```python
from build123d import *
from OCP.BRepFilletAPI import BRepFilletAPI_MakeChamfer

# Parameters (mm, degrees)
SKETCH1_W           = 251
SKETCH1_H           = 24.5
SKETCH1_W_2         = 243
SKETCH1_H_2         = 16.5
BOSS_EXTRUDE1_DEPTH = 25
SKETCH1_2_W         = 251
SKETCH1_2_H         = 24.5
BOSS_EXTRUDE2_DEPTH = 4
CHAMFER1_SIZE       = 10
CHAMFER1_SIZE2      = 1.763269807
FILLET1_R           = 10
FILLET2_R           = 1
FILLET4_R           = 10
FILLET5_R           = 5


with BuildPart() as part:
    # Sketch1 → Boss-Extrude1 (new body)
    with BuildSketch(Plane(origin=(0, 0, 0), x_dir=(1, 0, 0), z_dir=(0, 1, 0))):
        Rectangle(SKETCH1_W, SKETCH1_H)
        Rectangle(SKETCH1_W_2, SKETCH1_H_2, mode=Mode.SUBTRACT)
    extrude(amount=BOSS_EXTRUDE1_DEPTH)

    # Sketch1<2> → Boss-Extrude2 (add)
    with BuildSketch(Plane(origin=(0, 0, 0), x_dir=(1, 0, 0), z_dir=(0, 1, 0))):
        Rectangle(SKETCH1_2_W, SKETCH1_2_H)
    extrude(amount=-BOSS_EXTRUDE2_DEPTH)

    # Chamfer1: one chamfer whose edges measure the first distance from different faces: ONE call of the kernel's chamfer builder (chamfer() names one face for all edges)
    chamfer1_edges_1 = [part.edges().sort_by_distance(p)[0] for p in [
        (121.5, 12.5, 8.25),
        (0, 0, 8.25),
        (-121.5, 12.5, 8.25),
    ]]
    chamfer1_side_1 = [part.faces().sort_by_distance(p)[0] for p in [
        (0, 12.5, 8.25),
    ]]
    chamfer1_edges_2 = [part.edges().sort_by_distance(p)[0] for p in [
        (0, 0, -8.25),
        (121.5, 12.5, -8.25),
        (-121.5, 12.5, -8.25),
    ]]
    chamfer1_side_2 = [part.faces().sort_by_distance(p)[0] for p in [
        (0, 12.5, -8.25),
    ]]
    chamfer1 = BRepFilletAPI_MakeChamfer(part.part.solid().wrapped)
    for e in chamfer1_edges_1:
        chamfer1.Add(CHAMFER1_SIZE, CHAMFER1_SIZE2, e.wrapped, chamfer1_side_1[0].wrapped)  # the first distance lies on this face
    for e in chamfer1_edges_2:
        chamfer1.Add(CHAMFER1_SIZE, CHAMFER1_SIZE2, e.wrapped, chamfer1_side_2[0].wrapped)  # the first distance lies on this face
    add(Compound.cast(chamfer1.Shape()), mode=Mode.REPLACE)

    # Fillet1
    fillet1_edges = [part.edges().sort_by_distance(p)[0] for p in [
        (-111.5, 17.5, 8.25),
        (111.5, 17.5, 8.25),
        (111.5, 17.5, -8.25),
        (-111.5, 17.5, -8.25),
    ]]
    fillet(fillet1_edges, radius=FILLET1_R)

    # Fillet2
    fillet2_edges = [part.edges().sort_by_distance(p)[0] for p in [
        (121.5, 12.5, -6.486730193),
        (121.5, 12.5, 6.486730193),
        (-121.5, 12.5, -6.486730193),
        (-121.5, 12.5, 6.486730193),
    ]]
    fillet(fillet2_edges, radius=FILLET2_R)

    # Fillet4
    # the kernel refuses this fillet: 10 mm, written as the material it adds along each edge
    with BuildSketch(Plane(origin=(-121.5, 0, -30.647630562), x_dir=(0, 1, 0), z_dir=(0, 0, 1))) as fillet4_piece_1_section:
        with BuildLine():
            CenterArc((FILLET4_R, -FILLET4_R), FILLET4_R, 90, 90)
            Line((0, -FILLET4_R), (0, 0))
            Line((0, 0), (FILLET4_R, 0))
        make_face()
    fillet4_piece_1 = extrude(amount=61.295261123, mode=Mode.PRIVATE)
    fillet4_piece_1 = split(fillet4_piece_1, bisect_by=Plane(origin=(-119.266320611, 1.057029519, 6.673113017), z_dir=(0, 0.17364817766693139, -0.9848077530122079)), keep=Keep.TOP, mode=Mode.PRIVATE)
    fillet4_piece_1 = split(fillet4_piece_1, bisect_by=Plane(origin=(-119.266320611, 1.057029519, -6.673113017), z_dir=(0, 0.17364817766693139, 0.9848077530122079)), keep=Keep.TOP, mode=Mode.PRIVATE)
    add(fillet4_piece_1)
    with BuildSketch(Plane(origin=(121.5, 0, 30.647630562), x_dir=(0, 1, 0), z_dir=(0, 0, -1))) as fillet4_piece_2_section:
        with BuildLine():
            CenterArc((FILLET4_R, -FILLET4_R), FILLET4_R, 90, 90)
            Line((0, -FILLET4_R), (0, 0))
            Line((0, 0), (FILLET4_R, 0))
        make_face()
    fillet4_piece_2 = extrude(amount=61.295261123, mode=Mode.PRIVATE)
    fillet4_piece_2 = split(fillet4_piece_2, bisect_by=Plane(origin=(119.266320611, 1.057029519, 6.673113017), z_dir=(0, 0.17364817766693139, -0.9848077530122079)), keep=Keep.TOP, mode=Mode.PRIVATE)
    fillet4_piece_2 = split(fillet4_piece_2, bisect_by=Plane(origin=(119.266320611, 1.057029519, -6.673113017), z_dir=(0, 0.17364817766693139, 0.9848077530122079)), keep=Keep.TOP, mode=Mode.PRIVATE)
    add(fillet4_piece_2)

    # Fillet5
    fillet5_edges = [part.edges().sort_by_distance(p)[0] for p in [
        (-125.5, 10.5, -12.25),
        (125.5, 10.5, -12.25),
        (125.5, 10.5, 12.25),
        (-125.5, 10.5, 12.25),
    ]]
    fillet(fillet5_edges, radius=FILLET5_R)


solid = part.part
```
Check sheet for the modelled part. Datum: model origin and axes. Units: mm. A direction names the side the tool comes from. Round coordinates to 2 decimals unless told otherwise and drop trailing zeros. Write each loop counter-clockwise with the first axis right and the second up, starting at its lowest first coordinate (ties: lowest second). Pieces come first, ordered by that corner, then holes. Notation, with made-up numbers: (40.5, 4.5) -> (96.5, 4.5) arc R28 cw to (96.5, 41.5) -> close; hole circle Ø10 at (-28.5, 19). An arc over 180 degrees is marked (long way). Put each result on its own line as item: value.
(1) Go/stop test with a flat-tipped pin: pin 1 Ø6.5 at (x, z) = (-39, -2.5) entering from +Y. Record where the tip stops, or that it passes through.
Values found:
pin 1: stops at y = 0
(2) Sectioned sample at A-A (y = 22.5). Enter the section's corners in (x, z).
Values found:
outline: (-125.5, -7.25) arc R5 ccw to (-120.5, -12.25) -> (120.5, -12.25) arc R5 ccw to (125.5, -7.25) -> (125.5, 7.25) arc R5 ccw to (120.5, 12.25) -> (-120.5, 12.25) arc R5 ccw to (-125.5, 7.25) -> close; hole (-121.5, -5.65) arc R1 ccw to (-120.67, -6.63) -> (-112.36, -8.1) arc R10 ccw to (-110.63, -8.25) -> (110.63, -8.25) arc R10 ccw to (112.36, -8.1) -> (120.67, -6.63) arc R1 ccw to (121.5, -5.65) -> (121.5, 5.65) arc R1 ccw to (120.67, 6.63) -> (112.36, 8.1) arc R10 ccw to (110.63, 8.25) -> (-110.63, 8.25) arc R10 ccw to (-112.36, 8.1) -> (-120.67, 6.63) arc R1 ccw to (-121.5, 5.65) -> close
(3) Tool access check on faces 5 (the face through (-1, 25, 9)), 6 (the face through (118.65, 3.01, 0.1)). Record the directions out of +Z, -Z, +X, -X, +Y, -Y that give a thin tool (end or side, any length) a straight path to the whole face; none if there is none.
Values found:
face 5: +Z, -Z, +X, -X, +Y
face 6: +Y
(4) Sectioned sample at B-B (z = 2). Enter the section's corners in (x, y), plus the area to 3 significant figures.
Values found:
outline: (-125.5, -4) -> (125.5, -4) -> (125.5, 25) -> (121.5, 25) -> (121.5, 10) arc R10 cw to (111.5, 0) -> (-111.5, 0) arc R10 cw to (-121.5, 10) -> (-121.5, 25) -> (-125.5, 25) -> close
area: 1,250 mm^2
(5) Material ranges on line 1 (Z direction, x = -112.5, y = 10.75); line 2 (Z direction, x = -107, y = 21.25); line 3 (X direction, y = 14.5, z = -4.75), recorded low to high.
Values found:
line 1: z = -12.25 to -8.07, 8.07 to 12.25
line 2: z = -12.25 to -8.25, 8.25 to 12.25
line 3: x = -125.5 to -121.5, 121.5 to 125.5
(6) Mould release check, pull along Z, two halves, no side actions. Record for faces 1 (the face through (-2, 11, 12.25)), 2 (the face through (-1.66, 4.93, -7.356)), 3 (the face through (-124.07, 10.3, -10.75)), 4 (the face through (116.576, 16.262, 7.355)): released by +Z, released by -Z, zero draft, split by the parting line, or undercut.
Values found:
face 1: released by +Z
face 2: undercut
face 3: released by -Z
face 4: undercut
(7) Sectioned sample at C-C (x = -98). Enter the section's corners in (y, z).
Values found:
outline: (-4, -12.25) -> (25, -12.25) -> (25, -8.25) -> (10, -8.25) -> (0, -6.49) -> (0, 6.49) -> (10, 8.25) -> (25, 8.25) -> (25, 12.25) -> (-4, 12.25) -> close
